Input: part model. Units: mm. Frame: model coordinates. A direction names the side the tool comes from. Coordinates: 2 decimals unless noted, no trailing zeros. Write each loop counter-clockwise with the first axis right and the second up, starting at its lowest first coordinate (ties: lowest second). Pieces come first, ordered by that corner, then holes.
from build123d import *

# Parameters (mm, degrees)
CUT_EXTRUDE3_DEPTH      = 17.28
CUT_EXTRUDE3_DEPTH_BACK = 17.28
SKETCH3_R               = 1.125
CUT_EXTRUDE4_DEPTH      = 17.2800001
CIRPATTERN1_COUNT       = 3
FILLET4_R               = 2
SKETCH4_R               = 16.28
BOSS_EXTRUDE1_DEPTH     = 12.7
SKETCH5_R               = 1.6425
CUT_EXTRUDE5_DEPTH      = 50.7
CUT_EXTRUDE6_DEPTH      = 3.2004
CIRPATTERN2_COUNT       = 4
CIRPATTERN3_COUNT       = 4


with BuildPart() as part:
    # Sketch1 → Revolve1 (revolve)
    with BuildSketch(Plane.XY, mode=Mode.PRIVATE) as revolve1_sk:
        Polygon((9.14, 44), (12.89, 44), (12.89, 35.75), (16.28, 35.75), (16.28, 0), (12.53, 0), (12.53, 32), (9.14, 32), align=None)
    revolve(revolve1_sk.sketch.rotate(Axis((0, 0, 0), (0, 1, 0)), 90), axis=Axis((0, 0, 0), (0, 1, 0)))  # turned: the seam where the file's is

    # Sketch2 → Cut-Extrude3 (cut, two sides)
    with BuildSketch(Plane.XY) as cut_extrude3_sk:
        with BuildLine():
            Line((-8, 0), (8, 0))
            ThreePointArc((8, 0), (0, 8), (-8, 0))
        make_face()
    extrude(amount=CUT_EXTRUDE3_DEPTH, mode=Mode.SUBTRACT)
    extrude(cut_extrude3_sk.sketch, amount=-CUT_EXTRUDE3_DEPTH_BACK, mode=Mode.SUBTRACT)

    # Sketch3 → Cut-Extrude4 (cut, through all)
    with BuildSketch(Plane(origin=(0, 0, 0), x_dir=(0, 0, -1), z_dir=(1, 0, 0))):
        with Locations((0, 14.3)):
            Circle(SKETCH3_R)
    cut_extrude4 = extrude(amount=-CUT_EXTRUDE4_DEPTH, mode=Mode.SUBTRACT)

    # CirPattern1: Cut-Extrude4 ×3 about axis
    cirpattern1_axis = Axis((0, 46.725, 0), (0, -1, 0))
    for i in range(1, CIRPATTERN1_COUNT):
        add(cut_extrude4.rotate(cirpattern1_axis, i * 360 / CIRPATTERN1_COUNT), mode=Mode.SUBTRACT)

    # Fillet4
    fillet4_edges = [part.edges().sort_by_distance(p)[0] for p in [
        (0, 44, 12.89),
    ]]
    fillet(fillet4_edges, radius=FILLET4_R)

    # Sketch4 → Boss-Extrude1 (add)
    with BuildSketch(Plane(origin=(0, 35.75, 0), x_dir=(1, 0, 0), z_dir=(0, 1, 0))):
        with BuildLine():
            Line((-12.5, 48.102390793), (-12.5, 28.673827788))
            ThreePointArc((-12.5, 28.673827788), (-22.118300116, 22.118300116), (-28.673827788, 12.5))
            Line((-28.673827788, 12.5), (-48.102390793, 12.5))
            ThreePointArc((-48.102390793, 12.5), (-49.7, 0), (-48.102390793, -12.5))
            Line((-48.102390793, -12.5), (-28.673827788, -12.5))
            ThreePointArc((-28.673827788, -12.5), (-22.118300116, -22.118300116), (-12.5, -28.673827788))
            Line((-12.5, -28.673827788), (-12.5, -48.102390793))
            ThreePointArc((-12.5, -48.102390793), (0, -49.7), (12.5, -48.102390793))
            Line((12.5, -48.102390793), (12.5, -28.673827788))
            ThreePointArc((12.5, -28.673827788), (22.118300116, -22.118300116), (28.673827788, -12.5))
            Line((28.673827788, -12.5), (48.102390793, -12.5))
            ThreePointArc((48.102390793, -12.5), (49.7, 0), (48.102390793, 12.5))
            Line((48.102390793, 12.5), (28.673827788, 12.5))
            ThreePointArc((28.673827788, 12.5), (22.118300116, 22.118300116), (12.5, 28.673827788))
            Line((12.5, 28.673827788), (12.5, 48.102390793))
            ThreePointArc((12.5, 48.102390793), (0, 49.7), (-12.5, 48.102390793))
        make_face()
        with Locations(Location((0, 0, 0), (0, 0, 119.432673442))):  # turned: the seam where the file's is
            Circle(SKETCH4_R, mode=Mode.SUBTRACT)
    extrude(amount=-BOSS_EXTRUDE1_DEPTH)

    # Sketch5 → Cut-Extrude5 (cut, through all)
    with BuildSketch(Plane.XY):
        with Locations(Location((0, 29.4, 0), (0, 0, 90))):  # turned: the seam where the file's is
            Circle(SKETCH5_R)
    cut_extrude5 = extrude(amount=-CUT_EXTRUDE5_DEPTH, mode=Mode.SUBTRACT)

    # Sketch6 → Cut-Extrude6 (cut)
    with BuildSketch(Plane.XZ.offset(-23.05)):
        with BuildLine():
            Line((-12.5, 48.102390793), (-12.5, 46.007125807))
            ThreePointArc((-12.5, 46.007125807), (0, 47.675), (12.5, 46.007125807))
            Line((12.5, 46.007125807), (12.5, 48.102390793))
            ThreePointArc((12.5, 48.102390793), (0, 49.7), (-12.5, 48.102390793))
        make_face()
    cut_extrude6 = extrude(amount=-CUT_EXTRUDE6_DEPTH, mode=Mode.SUBTRACT)

    # CirPattern2: Cut-Extrude5 ×4 about axis
    cirpattern2_axis = Axis((0, 46.725, 0), (0, -1, 0))
    for i in range(1, CIRPATTERN2_COUNT):
        add(cut_extrude5.rotate(cirpattern2_axis, i * 360 / CIRPATTERN2_COUNT), mode=Mode.SUBTRACT)

    # CirPattern3: Cut-Extrude6 ×4 about axis
    cirpattern3_axis = Axis((0, 46.725, 0), (0, -1, 0))
    for i in range(1, CIRPATTERN3_COUNT):
        add(cut_extrude6.rotate(cirpattern3_axis, i * 360 / CIRPATTERN3_COUNT), mode=Mode.SUBTRACT)


solid = part.part
Item 1: Material intervals for line 1 (X direction, y = 29.4, z = 33.5); line 2 (Y direction, x = 29, z = 0), sorted ascending.
Item 2: Pin query (flat end, axial travel): pin 1 Ø4 at (x, z) = (-47.5, 1) entering from -Y; pin 2 Ø5 at (y, z) = (15.5, -12.5) entering from -X; pin 3 Ø4 at (x, y) = (-9.5, 15.5) entering from -Z; pin 4 Ø7.5 at (x, z) = (2, -4.5) entering from -Y. Return the tip coordinate at first contact, or that it passes through.
Item 3: Pull-direction query (X, two-part tool) for faces 4 (the face through (0, 8, -13)), 5 (the face through (-0.716, 11.364, 16.264)), 6 (the face through (47.675, 24.628, 0.177)); classes: released by +X, released by -X, zero draft, split by the parting line, or undercut.
Item 4: Access query for faces 1 (the face through (-0.177, 24.628, 47.675)), 2 (the face through (-47.675, 24.628, -0.177)), 3 (the face through (-12.5, 29, -39)). Directions: +Z, -Z, +X, -X, +Y, -Y. A direction counts if a zero-diameter tool reaches every point of the face in a straight line with its end or side. Return the directions, or none.
Item 5: Section query A-A, the plane y = 34. Return loops of the section in (x, z).
Item 6: Section query D-D, the plane y = 17.5. Return loops of the section in (x, z).
The answers:
1. line 1: x = -12.5 to -1.64, 1.64 to 12.5
1. line 2: y = 23.05 to 27.76, 31.04 to 35.75
2. pin 1: stops at y = 23.05
2. pin 2: stops at x = -12.85
2. pin 3: stops at z = -14.45
2. pin 4: passes through
3. face 4: undercut
3. face 5: split by the parting line
3. face 6: released by +X
4. face 1: +Z, -Y
4. face 2: -X, -Y
4. face 3: -Z, -X, +Y, -Y
5. outline: (-48.1, -12.5) - (-28.67, -12.5) arc R31.28 ccw to (-12.5, -28.67) - (-12.5, -48.1) arc R49.7 ccw to (12.5, -48.1) - (12.5, -28.67) arc R31.28 ccw to (28.67, -12.5) - (48.1, -12.5) arc R49.7 ccw to (48.1, 12.5) - (28.67, 12.5) arc R31.28 ccw to (12.5, 28.67) - (12.5, 48.1) arc R49.7 ccw to (-12.5, 48.1) - (-12.5, 28.67) arc R31.28 ccw to (-28.67, 12.5) - (-48.1, 12.5) arc R49.7 ccw to start; hole circle Ø18.28 at (0, 0)
6. outline: circle Ø32.56 at (0, 0); hole circle Ø25.06 at (0, 0)
